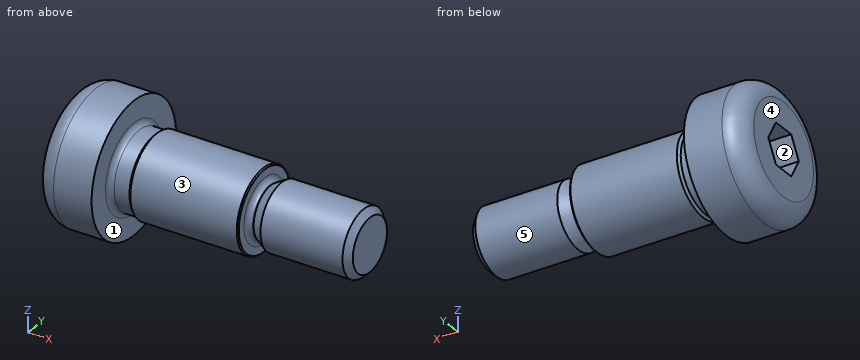
```python
from build123d import *

# Parameters (mm, degrees)
DODANIE_WYCI_GNI_CIE1_START       = -7
DODANIE_WYCI_GNI_CIE1_OUTLINE_R   = 8
DODANIE_WYCI_GNI_CIE1_DEPTH       = 7
DODANIE_WYCI_GNI_CIE1_START_2     = -1.133333233
DODANIE_WYCI_GNI_CIE1_2_OUTLINE_R = 4.71
DODANIE_WYCI_GNI_CIE1_2_DEPTH     = 3.633333233
SZKIC2_R                          = 4.71
DODANIE_WYCI_GNI_CIE2_DEPTH       = 0.29
DODANIE_WYCI_GNI_CIE2_DRAFT       = -45
SZKIC3_R                          = 5
DODANIE_WYCI_GNI_CIE3_DEPTH       = 13.11
SZKIC4_R                          = 3.2331875
DODANIE_WYCI_GNI_CIE4_DEPTH       = 0.7668125
SZKIC5_R                          = 3.2331875
DODANIE_WYCI_GNI_CIE5_DEPTH       = 1.32815821
DODANIE_WYCI_GNI_CIE5_DRAFT       = -30
SZKIC6_R                          = 4
DODANIE_WYCI_GNI_CIE6_DEPTH       = 10.76
SFAZOWANIE1_SIZE                  = 0.7668125
SFAZOWANIE2_SIZE                  = 0.15
ZAOKR_GLENIE1_R                   = 0.64
ZAOKR_GLENIE2_R                   = 2.3622


with BuildPart() as part:
    # Dodanie-wyciągnięcie1: read off the stored shape, not the designer's step
    # Dodanie-wyciągnięcie1 outline → Dodanie-wyciągnięcie1 (new body)
    with BuildSketch(Plane(origin=(0, 0, 0), x_dir=(0, 0, -1), z_dir=(1, 0, 0)).offset(DODANIE_WYCI_GNI_CIE1_START)):
        Circle(DODANIE_WYCI_GNI_CIE1_OUTLINE_R)
        Polygon((0, 2.886751346), (2.5, 1.443375673), (2.5, -1.443375673), (0, -2.886751346), (-2.5, -1.443375673), (-2.5, 1.443375673), align=None, mode=Mode.SUBTRACT)
    extrude(amount=DODANIE_WYCI_GNI_CIE1_DEPTH)

    # Dodanie-wyci_gni_cie1 2 outline → Dodanie-wyci_gni_cie1 2 (add)
    with BuildSketch(Plane(origin=(0, 0, 0), x_dir=(0, 0, -1), z_dir=(1, 0, 0)).offset(DODANIE_WYCI_GNI_CIE1_START_2)):
        Circle(DODANIE_WYCI_GNI_CIE1_2_OUTLINE_R)
    extrude(amount=DODANIE_WYCI_GNI_CIE1_2_DEPTH)

    # Dodanie-wyci_gni_cie1 3 outline → Dodanie-wyci_gni_cie1 3 (revolve)
    with BuildSketch(Plane.YX):
        Polygon((2.886751346, -1.133333233), (0, -1.133333233), (2.886751346, -2.8), align=None)
    revolve(axis=Axis((0, 0, 0), (1, 0, 0)))


with BuildPart() as dodanie_wyci_gni_cie2_tool:
    # Szkic2 → Dodanie-wyciągnięcie2 (with draft: the straight prism first)
    with BuildSketch(Plane(origin=(2.5, 0, 0), x_dir=(0, 0, -1), z_dir=(1, 0, 0))):
        with Locations(Location((0, 0, 0), (0, 0, 90))):
            Circle(SZKIC2_R)
    extrude(amount=DODANIE_WYCI_GNI_CIE2_DEPTH)
    # Dodanie-wyciągnięcie2: the draft: its side faces are tilted about the plane it starts from
    dodanie_wyci_gni_cie2_sides = [dodanie_wyci_gni_cie2_tool.faces().sort_by_distance(p)[0] for p in [
        (2.645, -4.71, 0),
    ]]
    draft(dodanie_wyci_gni_cie2_sides, Plane(origin=(2.5, 0, 0), x_dir=(0, 0, -1), z_dir=(1, 0, 0)), DODANIE_WYCI_GNI_CIE2_DRAFT)


with BuildPart() as part_1:
    add(part.part)

    # Dodanie-wyciągnięcie2: add dodanie_wyci_gni_cie2_tool
    add(dodanie_wyci_gni_cie2_tool.part)

    # Szkic3 → Dodanie-wyciągnięcie3 (add)
    with BuildSketch(Plane(origin=(2.79, 0, 0), x_dir=(0, 0, -1), z_dir=(1, 0, 0))):
        with Locations(Location((0, 0, 0), (0, 0, 270))):
            Circle(SZKIC3_R)
    extrude(amount=DODANIE_WYCI_GNI_CIE3_DEPTH)

    # Szkic4 → Dodanie-wyciągnięcie4 (add)
    with BuildSketch(Plane(origin=(15.9, 0, 0), x_dir=(0, 0, -1), z_dir=(1, 0, 0))):
        with Locations(Location((0, 0, 0), (0, 0, 270))):
            Circle(SZKIC4_R)
    extrude(amount=DODANIE_WYCI_GNI_CIE4_DEPTH)


with BuildPart() as dodanie_wyci_gni_cie5_tool:
    # Szkic5 → Dodanie-wyciągnięcie5 (with draft: the straight prism first)
    with BuildSketch(Plane(origin=(16.6668125, 0, 0), x_dir=(0, 0, -1), z_dir=(1, 0, 0))):
        with Locations(Location((0, 0, 0), (0, 0, 270))):
            Circle(SZKIC5_R)
    extrude(amount=DODANIE_WYCI_GNI_CIE5_DEPTH)
    # Dodanie-wyciągnięcie5: the draft: its side faces are tilted about the plane it starts from
    dodanie_wyci_gni_cie5_sides = [dodanie_wyci_gni_cie5_tool.faces().sort_by_distance(p)[0] for p in [
        (17.330891605, 3.2331875, 0),
    ]]
    draft(dodanie_wyci_gni_cie5_sides, Plane(origin=(16.6668125, 0, 0), x_dir=(0, 0, -1), z_dir=(1, 0, 0)), DODANIE_WYCI_GNI_CIE5_DRAFT)


with BuildPart() as part_2:
    add(part_1.part)

    # Dodanie-wyciągnięcie5: add dodanie_wyci_gni_cie5_tool
    add(dodanie_wyci_gni_cie5_tool.part)

    # Szkic6 → Dodanie-wyciągnięcie6 (add)
    with BuildSketch(Plane(origin=(17.99497071, 0, 0), x_dir=(0, 0, -1), z_dir=(1, 0, 0))):
        with Locations(Location((0, 0, 0), (0, 0, 90))):
            Circle(SZKIC6_R)
    extrude(amount=DODANIE_WYCI_GNI_CIE6_DEPTH)

    # Sfazowanie1
    sfazowanie1_edges = [part_2.edges().sort_by_distance(p)[0] for p in [
        (28.75497071, -4, 0),
    ]]
    chamfer(sfazowanie1_edges, length=SFAZOWANIE1_SIZE)

    # Sfazowanie2
    sfazowanie2_edges = [part_2.edges().sort_by_distance(p)[0] for p in [
        (15.9, 5, 0),
    ]]
    chamfer(sfazowanie2_edges, length=SFAZOWANIE2_SIZE)

    # Zaokrąglenie1
    zaokr_glenie1_edges = [part_2.edges().sort_by_distance(p)[0] for p in [
        (0, 0, 4.71),
        (15.9, 3.2331875, 0),
    ]]
    fillet(zaokr_glenie1_edges, radius=ZAOKR_GLENIE1_R)

    # Zaokrąglenie2
    zaokr_glenie2_edges = [part_2.edges().sort_by_distance(p)[0] for p in [
        (-7, 0, 8),
    ]]
    fillet(zaokr_glenie2_edges, radius=ZAOKR_GLENIE2_R)


solid = part_2.part
```
CAD build for the part. Positions are in the model's coordinates, mm. Face numbers are marked on the shaded views. A direction names the side the tool comes from. Coordinates: 2 decimals unless noted, no trailing zeros. Order: outer loops, then holes, each group sorted by start corner. A loop starts at its lowest first (then second) coordinate and runs counter-clockwise, first axis right, second up. Notation, with made-up numbers: (-22.75, 66) - (17.25, 66) arc R30 ccw to (17.25, 96) - close; hole circle Ø9 at (-12, -26.75). An arc over 180 degrees is marked (long way). Use a Markdown table: item, result. Add a question column.
(1) Which spindle directions (+Z, -Z, +X, -X, +Y, -Y) get a long thin tool onto all of the face, cutting with end or side? Do the marked faces 4 and 5. Say none if no direction does.
(2) Saw through at A-A (x = -2). Give the cut face in (y, z), then the cut area to 3 significant figures.
(3) Drill centre lines: line 1 along X through (y, z) = (2, -3); line 2 along X through (y, z) = (1.25, 4.25); line 3 along Z through (x, y) = (-3, -2). Where is each one in solid material? Low to high. Write a range as [from, to].
(4) Pull direction Z, two halves, no side cores. Call the marked faces 1, 2 and 3: +Z half, -Z half, draft (parallel to the pull), parting line (faces both ways), or undercut.
(5) Saw through at B-B (x = 14). Give the cut face in (y, z).
(6) Flat gauge pins, fed straight in: pin 1 (3 mm diameter, centred on x = 19, z = -0.5, fed in from +Y); pin 2 (1 mm diameter, centred on x = 24, y = -5, fed in from +Z); pin 3 (3 mm diameter, centred on x = 12, z = 0, fed in from -Y); pin 4 (5 mm diameter, centred on x = 5.5, z = -2.5, fed in from +Y). Where does each tip first touch, or does it go through?
Solved:
| question | item | result |
|---|---|---|
| 1 | face 4 | +Z, -Z, -X, +Y, -Y |
| 1 | face 5 | +X |
| 2 | outline | circle Ø16 at (0, 0); hole circle Ø3 at (0, 0) |
| 2 | area | 194 mm² |
| 3 | line 1 | x = [-7, 15.96], [17.31, 28.38] |
| 3 | line 2 | x = [-7, 15.9] |
| 3 | line 3 | z = [-7.75, -1.54], [1.54, 7.75] |
| 4 | face 1 | draft |
| 4 | face 2 | undercut |
| 4 | face 3 | parting line |
| 5 | outline | circle Ø10 at (0, 0) |
| 6 | pin 1 | stops at y = 4 |
| 6 | pin 2 | passes through |
| 6 | pin 3 | stops at y = -5 |
| 6 | pin 4 | stops at y = 5 |
